```python
from build123d import *

# Parameters (mm, degrees)
F6_DEPTH = 8
F7_DEPTH = 104
F8_START = 48
F8_DEPTH = 24


with BuildPart() as f6:
    # F5 (on Front) → F6 (new body)
    with BuildSketch(Plane.XZ):
        Polygon((258.1512545863, 8), (258.1512545863, 0), (720, 0), (720, -160), (256.8877548805, -474.8444829124), (123.8527919354, -474.8444829124), (96.8877548805, -474.8444829124), (103.7249146428, -461.4958824301), (103.7400223735, -461.4663866938), (103.8133779806, -461.3231701059), (103.8610917427, -461.2300156427), (257.951143964, -160.3906880696), (258.1512545863, -160), (249.0600389619, -157.1826700935), (246.6919749543, -164.824153775), (83.8018052429, -482.8444829124), (259.3496117054, -482.8444829124), (728, -164.234921787), (728, 8), align=None)
        Polygon((720, 0), (258.1512545863, 0), (258.1512545863, -160), (262.6014617103, -162.2793982877), (343.1600472217, -5), (715, -5), (715, -157.3531738831), (255.3490943649, -469.8444829124), (126.4137944058, -469.8444829124), (123.8527919354, -474.8444829124), (256.8877548805, -474.8444829124), (720, -160), align=None)
        Polygon((96.8877548805, -474.8444829124), (123.8527919354, -474.8444829124), (126.4137944058, -469.8444829124), (105.066473404, -469.8444829124), (108.2219495636, -463.6838559781), (106.4825408482, -462.7524437274), (103.7249146428, -461.4958824301), align=None)
        Polygon((279.3121381591, -171.3317998503), (262.401351088, -162.6700863573), (108.3112988667, -463.5094139303), (108.2795983128, -463.5713048387), (108.2219495636, -463.6838559781), (105.066473404, -469.8444829124), (126.4137944058, -469.8444829124), align=None)
        Polygon((262.6014617103, -162.2793982877), (258.1512545863, -160), (257.951143964, -160.3906880696), (262.401351088, -162.6700863573), align=None)
        Polygon((262.401351088, -162.6700863573), (257.951143964, -160.3906880696), (103.8610917427, -461.2300156427), (108.3112988667, -463.5094139303), align=None)
    extrude(amount=F6_DEPTH)

    # F5 (on Front) → F7 (join)
    with BuildSketch(Plane.XZ):
        Polygon((258.1512545863, 8), (258.1512545863, 0), (720, 0), (720, -160), (256.8877548805, -474.8444829124), (123.8527919354, -474.8444829124), (96.8877548805, -474.8444829124), (103.7249146428, -461.4958824301), (103.7400223735, -461.4663866938), (103.8133779806, -461.3231701059), (103.8610917427, -461.2300156427), (257.951143964, -160.3906880696), (258.1512545863, -160), (249.0600389619, -157.1826700935), (246.6919749543, -164.824153775), (83.8018052429, -482.8444829124), (259.3496117054, -482.8444829124), (728, -164.234921787), (728, 8), align=None)
    extrude(amount=F7_DEPTH)

    # F5 (on Front) → F8 (join)
    with BuildSketch(Plane.XZ.offset(F8_START)):
        Polygon((96.8877548805, -474.8444829124), (123.8527919354, -474.8444829124), (126.4137944058, -469.8444829124), (105.066473404, -469.8444829124), (108.2219495636, -463.6838559781), (106.4825408482, -462.7524437274), (103.7249146428, -461.4958824301), align=None)
        Polygon((279.3121381591, -171.3317998503), (262.401351088, -162.6700863573), (108.3112988667, -463.5094139303), (108.2795983128, -463.5713048387), (108.2219495636, -463.6838559781), (105.066473404, -469.8444829124), (126.4137944058, -469.8444829124), align=None)
    extrude(amount=F8_DEPTH)


solid = f6.part
```
For this review, take the finished solid that the model builds, in its own axes (mm). A direction names the side the tool comes from. Round coordinates to 2 decimals unless told otherwise and drop trailing zeros. Write each loop counter-clockwise with the first axis right and the second up, starting at its lowest first coordinate (ties: lowest second). Pieces come first, ordered by that corner, then holes.
1) Take a section at A-A on z = -27.5. Give the boundary of the cut face in (x, y).
Answer below:
outline: (258.15, -8) - (331.64, -8) - (331.64, 0) - (258.15, 0) - close; (715, -8) - (720, -8) - (720, -104) - (728, -104) - (728, 0) - (715, 0) - close
2) Mouldability with a two-part tool opening along X and no side actions: class faces 1 (the face through (166.387, -51.272, -321.608)), 2 (the face through (269, -8, -184)), 3 (the face through (486, -55, 0)) as +X half, -X half, draft (parallel to the pull), parting line (faces both ways), or undercut.
Answer below:
face 1: -X half
face 2: undercut
face 3: draft
3) Insertion check: pin 1 Ø1.5 at (y, z) = (-56, -227.5) entering from -X; pin 2 Ø12 at (x, y) = (240, -71) entering from +Z; pin 3 Ø1 at (x, y) = (641, -43) entering from -Z. Each pin has a flat end and moves straight along its axis. Give the tip position at first contact, or say it passes through.
Answer below:
pin 1: stops at x = 214.21
pin 2: stops at z = -166.18
pin 3: stops at z = -223.72
4) Take a section at C-C on y = -57. Give the boundary of the cut face in (x, z).
Answer below:
outline: (83.8, -482.84) - (259.35, -482.84) - (728, -164.23) - (728, 8) - (258.15, 8) - (258.15, 0) - (720, 0) - (720, -160) - (256.89, -474.84) - (123.85, -474.84) - (279.31, -171.33) - (262.4, -162.67) - (108.22, -463.68) - (106.48, -462.75) - (103.72, -461.5) - (258.15, -160) - (249.06, -157.18) - (246.69, -164.82) - close
5) Machinability: for faces 4 (the face through (201.79, -3.94, -322.68)), 5 (the face through (491.686, -55.328, -315.218)), 6 (the face through (194, -48, -318)), which of the approach directions +Z, -Z, +X, -X, +Y, -Y give a long, thin tool a straight path to every point of the face, cutting with its end or side? Answer none if there is none.
Answer below:
face 4: +Y, -Y
face 5: -Y
face 6: none
6) For line 1 along X through (y, z) = (-19.5, -129); line 2 along X through (y, z) = (-25, -386.5) (1 decimal); line 3 along X through (y, z) = (-84, -448.5), list the stretches that pass through material, from the lowest coordinate up.
Answer below:
line 1: x = 720 to 728
line 2: x = 133.1 to 142.1, 386.8 to 401.1
line 3: x = 101.39 to 110.38, 295.64 to 309.87
7) Take a section at B-B on x = 335. Give the boundary of the cut face in (y, z), then the cut area to 3 significant figures.
Answer below:
outline: (-104, -431.41) - (0, -431.41) - (0, -415.69) - (-8, -415.69) - (-8, -421.74) - (-104, -421.74) - close; (-104, 0) - (-8, 0) - (-8, -20.93) - (0, -20.93) - (0, 8) - (-104, 8) - close
area: 2,050 mm2
8) Take a section at D-D on z = -230.5. Give the boundary of the cut face in (x, y), then the cut area to 3 significant figures.
Answer below:
outline: (213.05, -104) - (222.04, -104) - (222.04, -8) - (249.01, -8) - (249.01, 0) - (213.05, 0) - close; (227.66, -72) - (249.01, -72) - (249.01, -48) - (227.66, -48) - close; (607.41, -8) - (616.3, -8) - (616.3, -104) - (630.53, -104) - (630.53, 0) - (607.41, 0) - close
area: 3,210 mm2
